from build123d import *

# Parameters (mm, degrees)
SKETCH1_R           = 49
SKETCH1_R_2         = 46
BOSS_EXTRUDE1_DEPTH = 10
SKETCH2_R           = 1.8
BOSS_EXTRUDE2_DEPTH = 3


with BuildPart() as part:
    # Sketch1 → Boss-Extrude1 (new body)
    with BuildSketch(Plane(origin=(0, 0, 0), x_dir=(1, 0, 0), z_dir=(0, 1, 0))):
        Circle(SKETCH1_R)
        Circle(SKETCH1_R_2, mode=Mode.SUBTRACT)
    extrude(amount=BOSS_EXTRUDE1_DEPTH)

    # Sketch2 → Boss-Extrude2 (add)
    with BuildSketch(Plane(origin=(0, 0, 0), x_dir=(1, 0, 0), z_dir=(0, 1, 0))):
        with BuildLine():
            Line((-46, 0), (-46, 4))
            Line((-46, 4), (-57, 4))
            ThreePointArc((-57, 4), (-58.414213562, 3.414213562), (-59, 2))
            Line((-59, 2), (-59, -2))
            ThreePointArc((-59, -2), (-58.414213562, -3.414213562), (-57, -4))
            Line((-57, -4), (-46, -4))
            Line((-46, -4), (-46, 0))
        make_face()
        with Locations((-54, 0)):
            Circle(SKETCH2_R, mode=Mode.SUBTRACT)
    boss_extrude2 = extrude(amount=BOSS_EXTRUDE2_DEPTH)

    # Mirror1: Boss-Extrude2 across plane
    add(boss_extrude2.mirror(Plane(origin=(0, 0, 0), x_dir=(0, 0, 1), z_dir=(1, 0, 0))))


solid = part.part
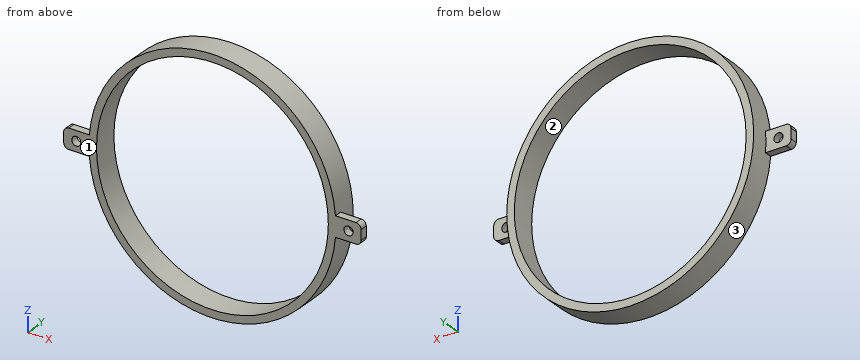
Here's how the part is built. I have some questions about the finished solid (model axes, mm). Face numbers are marked on the shaded views. Round coordinates to 2 decimals unless told otherwise and drop trailing zeros. Loops run counter-clockwise (first coordinate to the right, second up) from the corner with the lowest first, then second, coordinate; pieces in that order, holes last. Notation, with made-up numbers: (33.5, -38) - (44.5, -38) arc R28 ccw to (44.5, -19) - close; hole circle Ø1 at (36, 32). An arc over 180 degrees is marked (long way). One line per question, with ' | ' between items. Start each with the question number.
Q1. I want a section at C-C (z = -30.5). Write out the boundary of the cut face in (x, y).
Q2. Will these pins go through, and if not, where does the flat tip stop? pin 1 (1.5 mm diameter, centred on y = 8, z = 21.5, fed in from -X); pin 2 (6.5 mm diameter, centred on x = -54.5, z = 0, fed in from +Y); pin 3 (2.5 mm diameter, centred on x = 51, y = 1, fed in from -Z).
Q3. I want a section at D-D (y = 7.25). Write out the boundary of the cut face in (x, z), then the cut area to 3 significant figures.
Q4. We'd pull the mould along Z, two halves only. Please class the marked faces 1, 2 and 3: +Z half, -Z half, draft (parallel to the pull), parting line (faces both ways), or undercut.
Q5. Please list where these lines run through material, in increasing order: line 1 (X direction, y = 2.15, z = 0); line 2 (Z direction, x = -54, y = 2.3); line 3 (Z direction, x = 0, y = 7.5). Write a range as [from, to].
Q6. I want a section at B-B (x = 0). Write out the boundary of the cut face in (y, z).
Q7. I want a section at A-A (z = 0). Write out the boundary of the cut face in (x, y), then the cut area to 3 significant figures.
Response values:
1) outline: (-38.35, 0) - (-34.43, 0) - (-34.43, 10) - (-38.35, 10) - close; (34.43, 0) - (38.35, 0) - (38.35, 10) - (34.43, 10) - close
2) pin 1: stops at x = -44.39 | pin 2: stops at y = 3 | pin 3: stops at z = -4
3) outline: circle Ø98 at (0, 0); hole circle Ø92 at (0, 0) | area: 895 mm²
4) face 1: draft | face 2: undercut | face 3: parting line
5) line 1: x = [-59, -55.8], [-52.2, -46], [46, 52.2], [55.8, 59] | line 2: z = [-4, -1.8], [1.8, 4] | line 3: z = [-49, -46], [46, 49]
6) outline: (0, -49) - (10, -49) - (10, -46) - (0, -46) - close; (0, 46) - (10, 46) - (10, 49) - (0, 49) - close
7) outline: (-59, 0) - (-55.8, 0) - (-55.8, 3) - (-59, 3) - close; (-52.2, 0) - (-46, 0) - (-46, 10) - (-49, 10) - (-49, 3) - (-52.2, 3) - close; (46, 0) - (52.2, 0) - (52.2, 3) - (49, 3) - (49, 10) - (46, 10) - close; (55.8, 0) - (59, 0) - (59, 3) - (55.8, 3) - close | area: 98.4 mm²
